For this review, take the finished solid that the model builds, in its own axes (mm). A direction names the side the tool comes from. Round coordinates to 2 decimals unless told otherwise and drop trailing zeros. Write each loop counter-clockwise with the first axis right and the second up, starting at its lowest first coordinate (ties: lowest second). Pieces come first, ordered by that corner, then holes. Notation, with made-up numbers: M 17.25,-37.5 L 50.25,-37.5 A25 ccw 50.25,-9.5 Z; hole C 57,20 d11. An arc over 180 degrees is marked long. Answer in a Markdown table with one row per item.
```python
from build123d import *

# Parameters (mm, degrees)
F0_R     = 19.060581
F1_DEPTH = 1.5875
F2_R     = 3.494231
F3_DEPTH = 21.082
F4_R     = 3.237878
F5_DEPTH = 10.16
F6_R     = 1.655878
F7_DEPTH = 9.144


with BuildPart() as f1:
    # F0 (on Front) → F1 (new body)
    with BuildSketch(Plane.XZ):
        Circle(F0_R)
    extrude(amount=-F1_DEPTH)

    # F2 (on face) → F3 (cut)
    with BuildSketch(Plane.XZ):
        with Locations((0, 14.097)):
            Circle(F2_R)
        with Locations((-9.968085, 9.968085)):
            Circle(F2_R)
        with Locations((-14.097, 0)):
            Circle(F2_R)
        with Locations((-9.968085, -9.968085)):
            Circle(F2_R)
        with Locations((0, -14.097)):
            Circle(F2_R)
        with Locations((9.968085, -9.968085)):
            Circle(F2_R)
        with Locations((14.097, 0)):
            Circle(F2_R)
        with Locations((9.968085, 9.968085)):
            Circle(F2_R)
    extrude(amount=-F3_DEPTH, mode=Mode.SUBTRACT)

    # F4 (on Front) → F5 (join)
    with BuildSketch(Plane.XZ):
        Circle(F4_R)
    extrude(amount=-F5_DEPTH)

    # F6 (on face) → F7 (cut)
    with BuildSketch(Plane(origin=(0, 10.16, 0), x_dir=(-1, 0, 0), z_dir=(0, 1, 0))):
        Circle(F6_R)
    extrude(amount=-F7_DEPTH, mode=Mode.SUBTRACT)


solid = f1.part
```
Q1. Mouldability with a two-part tool opening along Z and no side actions: class faces 1 (the face through (0, 0, 0)), 2 (the face through (-10.764, 0.783, 1.05)), 3 (the face through (-15.126, 0.783, -11.598)) as +Z half, -Z half, draft (parallel to the pull), parting line (faces both ways), or undercut.
Found:
| item | result |
|---|---|
| face 1 | draft |
| face 2 | undercut |
| face 3 | parting line |
Q2. Machinability: for faces 4 (the face through (0, 1.016, 0)), 5 (the face through (-0.45, 0.78, -10.63)), which of the approach directions +Z, -Z, +X, -X, +Y, -Y give a long, thin tool a straight path to every point of the face, cutting with its end or side? Answer none if there is none.
Found:
| item | result |
|---|---|
| face 4 | +Y |
| face 5 | +Y, -Y |
Q3. For probe 1 along Z at (x, y) = (0, 0.3); probe 2 along X at (y, z) = (1.5, -11); probe 3 along Y at (x, z) = (-4, 4), list the stretches that pass through material, from the lowest coordinate up.
Found:
| item | result |
|---|---|
| probe 1 | -19.06 to -17.59, -10.6 to 10.6, 17.59 to 19.06 |
| probe 2 | -15.57 to -13.31, -6.63 to -1.62, 1.62 to 6.63, 13.31 to 15.57 |
| probe 3 | 0 to 1.59 |
Q4. Take a section at A-A (x = 0). State the section outline as (y, z) points, then the cut area to 3 significant figures.
Found:
| item | result |
|---|---|
| outline | M 0,-19.06 L 1.59,-19.06 L 1.59,-17.59 L 0,-17.59 Z; M 0,-10.6 L 1.59,-10.6 L 1.59,-3.24 L 10.16,-3.24 L 10.16,-1.66 L 1.02,-1.66 L 1.02,1.66 L 10.16,1.66 L 10.16,3.24 L 1.59,3.24 L 1.59,10.6 L 0,10.6 Z; M 0,17.59 L 1.59,17.59 L 1.59,19.06 L 0,19.06 Z |
| area | 63.6 mm² |
Q5. Insertion check: P1, Ø3, axis at x = 10.5, y = 5, coming from the -Z side; P2, Ø9, axis at x = 0, z = -14.097, coming from the +Y side. Each pin has a flat end and moves straight along its axis. Give the tip position at first contact, or say it passes through.
Found:
| item | result |
|---|---|
| P1 | through |
| P2 | y = 1.59 |
Q6. Take a section at C-C (z = 11.5). State the section outline as (x, y) points, then the cut area to 3 significant figures.
Found:
| item | result |
|---|---|
| outline | M -15.2,0 L -13.11,0 L -13.11,1.59 L -15.2,1.59 Z; M -6.83,0 L -2.34,0 L -2.34,1.59 L -6.83,1.59 Z; M 2.34,0 L 6.83,0 L 6.83,1.59 L 2.34,1.59 Z; M 13.11,0 L 15.2,0 L 15.2,1.59 L 13.11,1.59 Z |
| area | 20.9 mm² |
Q7. Take a section at D-D (y = 2.25). State the section outline as (x, z) points.
Found:
| item | result |
|---|---|
| outline | C 0,0 d6.48; hole C 0,0 d3.31 |
Q8. Take a section at B-B (z = 0). State the section outline as (x, y) points.
Found:
| item | result |
|---|---|
| outline | M -19.06,0 L -17.59,0 L -17.59,1.59 L -19.06,1.59 Z; M -10.6,0 L 10.6,0 L 10.6,1.59 L 3.24,1.59 L 3.24,10.16 L 1.66,10.16 L 1.66,1.02 L -1.66,1.02 L -1.66,10.16 L -3.24,10.16 L -3.24,1.59 L -10.6,1.59 Z; M 17.59,0 L 19.06,0 L 19.06,1.59 L 17.59,1.59 Z |
